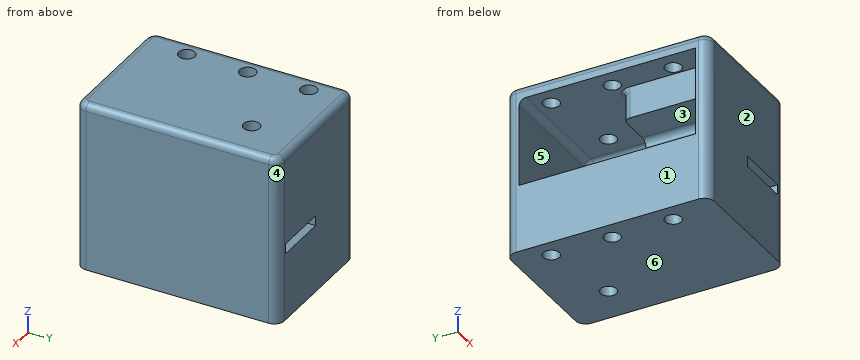
from build123d import *

# Parameters (mm, degrees)
SKETCH1_W               = 20
SKETCH1_H               = 30
BOSS_EXTRUDE1_DEPTH     = 25
CUT_EXTRUDE2_DEPTH      = 44.874821937
CUT_EXTRUDE2_DEPTH_BACK = 44.874821937
SKETCH4_W               = 8
SKETCH4_H               = 1.5
SKETCH5_W               = 8
SKETCH5_H               = 11.5
CUT_EXTRUDE3_DEPTH      = 15
SKETCH6_W               = 6.664038992
SKETCH6_H               = 13
CUT_EXTRUDE4_DEPTH      = 28
SKETCH7_W               = 8
SKETCH7_H               = 9
CUT_EXTRUDE5_DEPTH      = 3
SKETCH11_W              = 6.664038992
SKETCH11_H              = 2
BOSS_EXTRUDE2_DEPTH     = 13
SKETCH12_W              = 8
SKETCH12_H              = 2
BOSS_EXTRUDE3_DEPTH     = 11.5
SKETCH13_W              = 13
SKETCH13_H              = 26
CUT_EXTRUDE7_DEPTH      = 4
SKETCH18_R              = 1.2
CUT_EXTRUDE8_DEPTH      = 44.874821937
LPATTERN1_COUNT         = 3
LPATTERN1_PITCH         = 9
SKETCH19_W              = 4.7
SKETCH19_H              = 13
BOSS_EXTRUDE5_DEPTH     = 6
FILLET1_R               = 1.5
FILLET2_R               = 1
FILLET3_R               = 1
FILLET4_R               = 1
FILLET5_R               = 1
FILLET6_R               = 1
FILLET7_R               = 1
FILLET8_R               = 1
FILLET9_R               = 1
FILLET11_R              = 1
SKETCH20_R              = 1.2
CUT_EXTRUDE9_DEPTH      = 44.874821937


with BuildPart() as part:
    # Sketch1 → Boss-Extrude1 (new body)
    with BuildSketch(Plane.XY):
        with Locations((10, -15)):
            Rectangle(SKETCH1_W, SKETCH1_H)
    extrude(amount=BOSS_EXTRUDE1_DEPTH)

    # Sketch4 → Cut-Extrude2 (cut, two sides: drawn at the far end of the back side and taken through both)
    with BuildSketch(Plane.XZ.offset(30).offset(-CUT_EXTRUDE2_DEPTH_BACK)):
        with Locations((14.251880329, 10.75)):
            Rectangle(SKETCH4_W, SKETCH4_H)
    extrude(amount=CUT_EXTRUDE2_DEPTH + CUT_EXTRUDE2_DEPTH_BACK, mode=Mode.SUBTRACT)

    # Sketch5 → Cut-Extrude3 (cut)
    with BuildSketch(Plane(origin=(0, 0, 0), x_dir=(1, 0, 0), z_dir=(0, 1, 0))):
        with Locations((14.251880329, -17.25)):
            Rectangle(SKETCH5_W, SKETCH5_H)
    extrude(amount=-CUT_EXTRUDE3_DEPTH, mode=Mode.SUBTRACT)

    # Sketch6 → Cut-Extrude4 (cut)
    with BuildSketch(Plane.XZ.offset(30)):
        with Locations((6.919860833, 16.5)):
            Rectangle(SKETCH6_W, SKETCH6_H)
    extrude(amount=-CUT_EXTRUDE4_DEPTH, mode=Mode.SUBTRACT)

    # Sketch7 → Cut-Extrude5 (cut)
    with BuildSketch(Plane.XY.offset(10)):
        with Locations((14.251880329, -7.5)):
            Rectangle(SKETCH7_W, SKETCH7_H)
    extrude(amount=-CUT_EXTRUDE5_DEPTH, mode=Mode.SUBTRACT)

    # Sketch11 → Boss-Extrude2 (add)
    with BuildSketch(Plane.XY.offset(10)):
        with Locations((6.919860833, -29)):
            Rectangle(SKETCH11_W, SKETCH11_H)
    extrude(amount=BOSS_EXTRUDE2_DEPTH)

    # Sketch12 → Boss-Extrude3 (add)
    with BuildSketch(Plane(origin=(0, 0, 23), x_dir=(-1, 0, 0), z_dir=(0, 0, -1))):
        with Locations((-14.251880329, -1)):
            Rectangle(SKETCH12_W, SKETCH12_H)
    extrude(amount=BOSS_EXTRUDE3_DEPTH)

    # Sketch13 → Cut-Extrude7 (cut)
    with BuildSketch(Plane.ZY):
        with Locations((16.5, -15)):
            Rectangle(SKETCH13_W, SKETCH13_H)
    extrude(amount=-CUT_EXTRUDE7_DEPTH, mode=Mode.SUBTRACT)

    # Sketch18 → Cut-Extrude8 (cut, symmetric)
    with BuildSketch(Plane(origin=(0, 0, 0), x_dir=(-1, 0, 0), z_dir=(0, 0, -1))):
        with Locations((-2.8, -23.174436274)):
            Circle(SKETCH18_R)
    cut_extrude8 = extrude(amount=CUT_EXTRUDE8_DEPTH, both=True, mode=Mode.SUBTRACT)

    # LPattern1: Cut-Extrude8 ×3
    with Locations(*[(0, i * LPATTERN1_PITCH, 0) for i in range(1, LPATTERN1_COUNT)]):
        add(cut_extrude8, mode=Mode.SUBTRACT)

    # Sketch19 → Boss-Extrude5 (add)
    with BuildSketch(Plane.ZY.offset(-10.251880329)):
        with Locations((20.65, -21.5)):
            Rectangle(SKETCH19_W, SKETCH19_H)
    extrude(amount=BOSS_EXTRUDE5_DEPTH)

    # Fillet1
    fillet1_edges = [part.edges().sort_by_distance(p)[0] for p in [
        (20, 0, 12.5),
        (20, -30, 12.5),
        (0, -30, 12.5),
        (0, 0, 12.5),
    ]]
    fillet(fillet1_edges, radius=FILLET1_R)

    # Fillet2
    fillet2_edges = [part.edges().sort_by_distance(p)[0] for p in [
        (10.251880329, -21.5, 18.3),
    ]]
    fillet(fillet2_edges, radius=FILLET2_R)

    # Fillet3
    fillet3_edges = [part.edges().sort_by_distance(p)[0] for p in [
        (10.251880329, -7.5, 10),
    ]]
    fillet(fillet3_edges, radius=FILLET3_R)

    # Fillet4
    fillet4_edges = [part.edges().sort_by_distance(p)[0] for p in [
        (18.251880329, -8.5, 23),
    ]]
    fillet(fillet4_edges, radius=FILLET4_R)

    # Fillet5
    fillet5_edges = [part.edges().sort_by_distance(p)[0] for p in [
        (10, 0, 25),
        (20, -15, 25),
        (0, -15, 25),
        (10, -30, 25),
        (0.439339828, -29.560660172, 25),
        (19.560660172, -29.560660172, 25),
        (0.439339828, -0.439339828, 25),
        (19.560660172, -0.439339828, 25),
    ]]
    fillet(fillet5_edges, radius=FILLET5_R)

    # Fillet6
    fillet6_edges = [part.edges().sort_by_distance(p)[0] for p in [
        (18.251880329, -7.5, 7),
        (10.251880329, -7.5, 7),
    ]]
    fillet(fillet6_edges, radius=FILLET6_R)

    # Fillet7
    fillet7_edges = [part.edges().sort_by_distance(p)[0] for p in [
        (18.251880329, -15, 16.75),
        (17.95898711, -15, 22.707106781),
        (10.751880329, -15, 23),
    ]]
    fillet(fillet7_edges, radius=FILLET7_R)

    # Fillet8
    fillet8_edges = [part.edges().sort_by_distance(p)[0] for p in [
        (8.625940164, -2, 23),
        (17.95898711, -2, 22.707106781),
        (18.251880329, -2, 16.75),
    ]]
    fillet(fillet8_edges, radius=FILLET8_R)

    # Fillet9
    # the kernel refuses this fillet: 1 mm, written as the material it takes off along each edge
    with BuildSketch(Plane(origin=(4.251880329, -15, 22), x_dir=(0, -1, 0), z_dir=(0, 0, -1))) as fillet9_piece_1:
        with BuildLine():
            CenterArc((FILLET9_R, -FILLET9_R), FILLET9_R, 90, 90)
            Line((0, -FILLET9_R), (0, 0))
            Line((0, 0), (FILLET9_R, 0))
        make_face()
    extrude(amount=6.2, mode=Mode.SUBTRACT)
    with BuildSketch(Plane(origin=(4.251880329, -14, 22), x_dir=(0, 0.5976672776328242, -0.8017442392976507), z_dir=(0, -0.8017442392976507, -0.5976672776328242))) as fillet9_piece_2_section:
        with BuildLine():
            CenterArc((1 + FILLET9_R, FILLET9_R), FILLET9_R, 180, 90)
            Line((1 + FILLET9_R, 0), (1, 0))
            Line((1, 0), (1, FILLET9_R))
        make_face()
    fillet9_piece_2 = revolve(axis=Axis((4.251880329, -14, 22), (1, 0, 0)), revolution_arc=233.296989237, mode=Mode.PRIVATE)
    fillet9_piece_2 = split(fillet9_piece_2, bisect_by=Plane(origin=(4.563508846, -14.749938848, 23), z_dir=(0, 0, -1)), keep=Keep.TOP, mode=Mode.PRIVATE)
    add(fillet9_piece_2, mode=Mode.SUBTRACT)

    # Fillet11
    fillet11_edges = [part.edges().sort_by_distance(p)[0] for p in [
        (4.251880329, -28, 20.65),
    ]]
    fillet(fillet11_edges, radius=FILLET11_R)

    # Sketch20 → Cut-Extrude9 (cut, through all)
    with BuildSketch(Plane.XY.offset(25)):
        with Locations((14.161317573, -7.269489093)):
            Circle(SKETCH20_R)
    extrude(amount=-CUT_EXTRUDE9_DEPTH, mode=Mode.SUBTRACT)


solid = part.part
CAD build for the part. Positions are in the model's coordinates, mm. Face numbers are marked on the shaded views. A direction names the side the tool comes from. Round coordinates to 2 decimals unless told otherwise and drop trailing zeros. Write each loop counter-clockwise with the first axis right and the second up, starting at its lowest first coordinate (ties: lowest second). Pieces come first, ordered by that corner, then holes. Notation, with made-up numbers: M -13.75,37 L -6.75,37 A20 cw -6.75,73 Z; hole C 54.25,78 d4. An arc over 180 degrees is marked long. Put each result on its own line as item: value. Start each with the question number.
1) Pull direction Y, two halves, no side cores. Call the marked faces 1, 2, 3 and 4: pulls with the +Y half, pulls with the -Y half, needs draft (parallel to the pull), parting line crosses it, or undercut.
2) 3-axis set-ups, long thin cutter, end or side, ignore diameter. For the marked faces 5 and 6: which of +Z, -Z, +X, -X, +Y, -Y reach the whole face in a straight line?
3) Saw through at C-C, the plane y = -20.25. Write the cut outline in (x, z), and give its area (3 significant figures).
4) Saw through at B-B, the plane x = 6.5. Write the cut outline in (y, z), and give its area (3 significant figures).
5) Drill centre lines: probe 1 along Y at (x, z) = (2.8, 6.25); probe 2 along Z at (x, y) = (5, -10.75); probe 3 along X at (y, z) = (-14.25, 6.25). Where is each one in solid material? Low to high. Write a range as [from, to].
6) Saw through at A-A, the plane z = 10.5. Write the cut outline in (x, y).
7) Saw through at D-D, the plane x = 2.8. Count the separate pieces of the cut face and the enclosed holes in it, and give its area (3 significant figures).
8) Pin check, flat tip, straight feed: pin 1 Ø9 at (x, y) = (14, -22) entering from -Z. Stop position of the tip, or through.
Resolved:
1. face 1: needs draft
1. face 2: pulls with the -Y half
1. face 3: undercut
1. face 4: pulls with the +Y half
2. face 5: -X
2. face 6: -Z, +X, -X, +Y, -Y
3. outline: M 0,0 L 20,0 L 20,24 A1 ccw 19,25 L 1,25 A1 ccw 0,24 L 0,23 L 4.25,23 L 4.25,18.3 L 9.25,18.3 A1 cw 10.25,17.3 L 10.25,11.5 L 18.25,11.5 L 18.25,10 L 0,10 Z
3. area: 383 mm²
4. outline: M -30,0 L 0,0 L 0,24 A1 ccw -1,25 L -29,25 A1 ccw -30,24 Z; hole M -28,10 L -2,10 L -2,22 A1 ccw -3,23 L -14,23 A1 ccw -15,22 L -15,18.3 L -28,18.3 Z
4. area: 473 mm²
5. probe 1: [-30, -24.37], [-21.97, -15.37], [-12.97, -6.37], [-3.97, 0]
5. probe 2: [0, 10], [23, 25]
5. probe 3: [0, 1.6], [4, 20]
6. outline: M 0,-28.5 A1.5 ccw 1.5,-30 L 10.25,-30 L 10.25,-28 L 0,-28 Z; M 0,-2 L 10.25,-2 L 10.25,0 L 1.5,0 A1.5 ccw 0,-1.5 Z; M 18.25,-30 L 18.5,-30 A1.5 ccw 20,-28.5 L 20,-1.5 A1.5 ccw 18.5,0 L 18.25,0 Z
7. separate pieces: 6
7. enclosed holes: 0
7. area: 325 mm²
8. pin 1: z = 0
